Input: part model. Units: mm. Frame: model coordinates. A direction names the side the tool comes from. Coordinates: 2 decimals unless noted, no trailing zeros. Loops run counter-clockwise (first coordinate to the right, second up) from the corner with the lowest first, then second, coordinate; pieces in that order, holes last. Notation, with made-up numbers: M 67.25,32.5 L 89.25,32.5 A37 ccw 89.25,68.5 Z; hole C 31,32.25 d6. An arc over 180 degrees is marked long. Use a Markdown table: item, result. Add a question column.
1. Section B-B on x = -20.32. Output: boundary loops of the cut face in (y, z).
2. Pin query (flat end, axial travel): pin 1 (2.5 mm diameter, centred on x = -20.32, z = -15.875, fed in from -Y). Return the tip coordinate at first contact, or that it passes through.
3. Section C-C on y = 1.15. Output: boundary loops of the cut face in (x, z) (3 decimals).
4. Section A-A on z = 0. Output: boundary loops of the cut face in (x, y) (3 decimals).
5. Draft query along X for faces 1 (the flat face through (-13, 2, -19.05)), 2 (the flat face through (0, 2, 0)), 3 (the cylindrical face through (-6.25, 1.53, 16.77)). Return one class per face: +X half, -X half, draft (parallel to the pull), parting line (faces both ways), or undercut.
6. Set-up query: faces 4 (the flat face through (-13, 3.099, -13)), 5 (the flat face through (-22.225, 2, 0)). Return all of +Z, -Z, +X, -X, +Y, -Y with unobstructed straight access to the full face (end or side cutting, diameter ignored); none if empty.
7. Line query: L1, parallel to Z at x = -20.32, y = 0.8; L2, parallel to X at y = 0.45, z = 3.5 (3 decimals); L3, parallel to Z at x = -16, y = 2.4. Output: solid intervals per line, ascending. Write a range as [from, to].
```python
from build123d import *

# Parameters (mm, degrees)
SKETCH1_W           = 25.4
SKETCH1_H           = 38.1
SKETCH1_R           = 1.4732
SKETCH1_W_2         = 19.05
SKETCH1_H_2         = 25.4
BOSS_EXTRUDE1_DEPTH = 3.0988


with BuildPart() as part:
    # Sketch1 → Boss-Extrude1 (new body)
    with BuildSketch(Plane(origin=(0, 0, 0), x_dir=(1, 0, 0), z_dir=(0, 1, 0))):
        with Locations((-12.7, 0)):
            Rectangle(SKETCH1_W, SKETCH1_H)
        with Locations((-5.08, 15.875)):
            Circle(SKETCH1_R, mode=Mode.SUBTRACT)
        with Locations((-20.32, -15.875)):
            Circle(SKETCH1_R, mode=Mode.SUBTRACT)
        with Locations((-20.32, 15.875)):
            Circle(SKETCH1_R, mode=Mode.SUBTRACT)
        with Locations((-5.08, -15.875)):
            Circle(SKETCH1_R, mode=Mode.SUBTRACT)
        with Locations((-12.7, 0)):
            Rectangle(SKETCH1_W_2, SKETCH1_H_2, mode=Mode.SUBTRACT)
    extrude(amount=BOSS_EXTRUDE1_DEPTH)


solid = part.part
```
Answers below:
| question | item | result |
|---|---|---|
| 1 | outline | M 0,-19.05 L 3.1,-19.05 L 3.1,-17.35 L 0,-17.35 Z; M 0,-14.4 L 3.1,-14.4 L 3.1,-12.7 L 0,-12.7 Z; M 0,12.7 L 3.1,12.7 L 3.1,14.4 L 0,14.4 Z; M 0,17.35 L 3.1,17.35 L 3.1,19.05 L 0,19.05 Z |
| 2 | pin 1 | passes through |
| 3 | outline | M -25.4,-19.05 L 0,-19.05 L 0,19.05 L -25.4,19.05 Z; hole M -22.225,-12.7 L -3.175,-12.7 L -3.175,12.7 L -22.225,12.7 Z; hole C -20.32,-15.875 d2.946; hole C -20.32,15.875 d2.946; hole C -5.08,-15.875 d2.946; hole C -5.08,15.875 d2.946 |
| 4 | outline | M -25.4,0 L -22.225,0 L -22.225,3.099 L -25.4,3.099 Z; M -3.175,0 L 0,0 L 0,3.099 L -3.175,3.099 Z |
| 5 | face 1 | draft |
| 5 | face 2 | +X half |
| 5 | face 3 | undercut |
| 6 | face 4 | +Z, -Z, +X, -X, +Y |
| 6 | face 5 | +Y, -Y |
| 7 | L1 | z = [-19.05, -17.35], [-14.4, -12.7], [12.7, 14.4], [17.35, 19.05] |
| 7 | L2 | x = [-25.4, -22.225], [-3.175, 0] |
| 7 | L3 | z = [-19.05, -12.7], [12.7, 19.05] |
